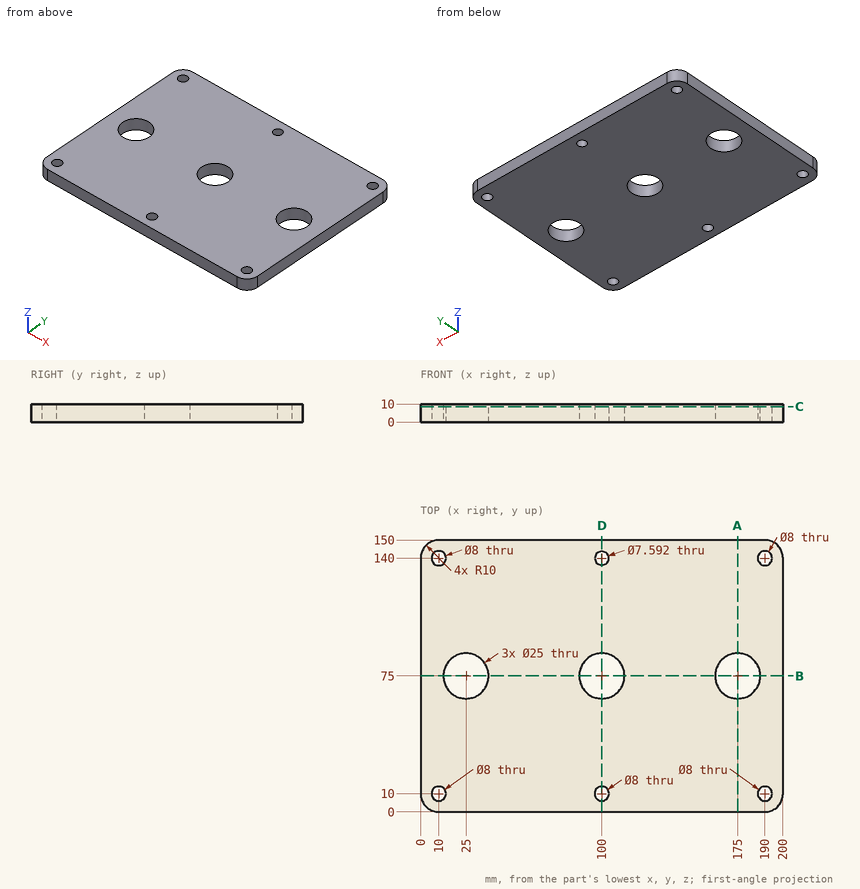
Can you work these out from the drawing? Everything is in mm from the part's minimum corner. Give positions to 0.01 mm unless a question says otherwise; leave off trailing zeros. Write each loop counter-clockwise with the first axis right and the second up, starting at its lowest first coordinate (ties: lowest second). Pieces come first, ordered by that corner, then holes. Notation, with made-up numbers: M 16.25,-38 L 40.25,-38 A20 ccw 40.25,-16 Z; hole C -4,55 d2. An arc over 180 degrees is marked long. Answer in a Markdown table with one row per item. Add a question column.
Item 1: Imagine slicing it at C-C, the plane z = 8.5. State how many separate pieces and enclosed holes the cut face has, plus the area to 3 significant figures.
Item 2: For pin 1 Ø5 at (x, y) = (190, 140) entering from -Z, with a flat end and sliding along its axis, tell me the tip position at first contact or that it passes through.
Item 3: Imagine slicing it at B-B, the plane y = 75. Write out the boundary of the cut face in (x, z), plus the area to 3 significant figures.
Item 4: Please list where these lines run through material, in increasing order: L1, parallel to Y at x = 100, z = 7.75; L2, parallel to Y at x = 175, z = 4.75; L3, parallel to X at y = 70.5, z = 8.5.
Item 5: Imagine slicing it at A-A, the plane x = 175. Write out the boundary of the cut face in (y, z), plus the area to 3 significant figures.
Item 6: Imagine slicing it at D-D, the plane x = 100. Write out the boundary of the cut face in (y, z), plus the area to 3 significant figures.
Evaluation:
| question | item | result |
|---|---|---|
| 1 | separate pieces | 1 |
| 1 | enclosed holes | 9 |
| 1 | area | 28,100 mm² |
| 2 | pin 1 | passes through |
| 3 | outline | M 0,0 L 12.5,0 L 12.5,10 L 0,10 Z; M 37.5,0 L 87.5,0 L 87.5,10 L 37.5,10 Z; M 112.5,0 L 162.5,0 L 162.5,10 L 112.5,10 Z; M 187.5,0 L 200,0 L 200,10 L 187.5,10 Z |
| 3 | area | 1,250 mm² |
| 4 | L1 | y = 0 to 6, 14 to 62.5, 87.5 to 136.2, 143.8 to 150 |
| 4 | L2 | y = 0 to 62.5, 87.5 to 150 |
| 4 | L3 | x = 0 to 13.34, 36.66 to 88.34, 111.66 to 163.34, 186.66 to 200 |
| 5 | outline | M 0,0 L 62.5,0 L 62.5,10 L 0,10 Z; M 87.5,0 L 150,0 L 150,10 L 87.5,10 Z |
| 5 | area | 1,250 mm² |
| 6 | outline | M 0,0 L 6,0 L 6,10 L 0,10 Z; M 14,0 L 62.5,0 L 62.5,10 L 14,10 Z; M 87.5,0 L 136.2,0 L 136.2,10 L 87.5,10 Z; M 143.8,0 L 150,0 L 150,10 L 143.8,10 Z |
| 6 | area | 1,090 mm² |
